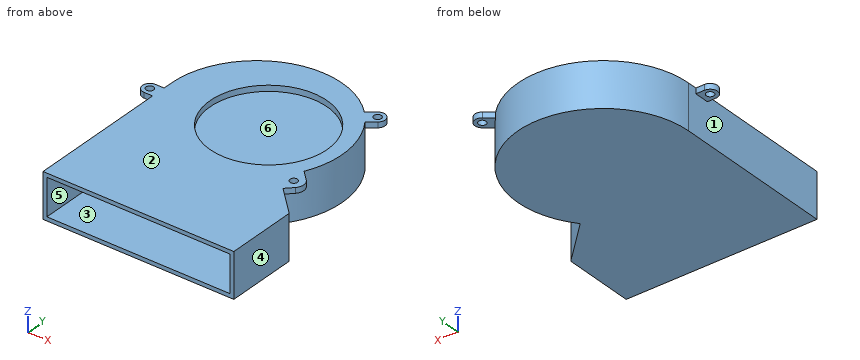
Autodesk Fusion 360 part; units mm, degrees
sketch "Esquisse1" plane through (0, 0, 0) normal (0, 0, 1) x (1, 0, 0)
  line L0 (0, 0) -> (98.3, 0)
  line L1 (98.3, 0) -> (98.3, 36.6)
  line L2 (98.3, 36.6) -> (77.8168, 56.6)
  arc A0 (77.8168, 56.6) -> (0, 84.75) centre (44, 84.75) ccw
  line L3 (0, 84.75) -> (0, 0)
  circle A1 centre (50.69, 84) radius 30.15
  point P0 (44, 128.75)
  point P1 (80.84, 84)
  point P2 (88, 84.75)
  point P3 (50.69, 114.15)
  dimension "d1" = 98.3
  dimension "d2" = 36.6
  dimension "d3" = 128.75
  dimension "d4" = 44
  dimension "d5" = 56.6
  dimension "d6" = 60.3
  dimension "d23" = 7.16
  dimension "d24" = 14.6
extrude "Extrusion1" add sketch "Esquisse1" along normal blind 23.06 contours L0 L1 L2 A0 L3 | A1
extrude "Extrusion2" cut sketch "Esquisse1" against normal blind 3 from surface at 23.06 contours A1
shell "Coque1" thickness 2 removed faces 1 at (32.7667, 0, 7.6867)
ref_plane "Plan de construction1" through (49.3725, 68.154, 23.06) normal (0, 0, 1) x (1, 0, 0)
sketch "Esquisse2" plane through (0, 0, 23.06) normal (0, 0, 1) x (1, 0, 0)
  circle A0 centre (84.6158, 57.1208) radius 1.95
  circle A1 centre (81.8543, 116.0561) radius 1.95
  circle A2 centre (-4.3677, 76.1716) radius 1.95
  line L0 (81.8543, 116.0561) -> (84.6158, 57.1208) construction
  line L1 (84.6158, 57.1208) -> (-4.3677, 76.1716) construction
  line L2 (81.8543, 116.0561) -> (-4.3677, 76.1716) construction
  circle A3 centre (44, 84.75) radius 49.1225 construction
  arc A4 (77.8168, 56.6) -> (0, 84.75) centre (44, 84.75) ccw construction
  circle A5 centre (84.6158, 57.1208) radius 5.1225
  line L3 (98.3, 36.6) -> (77.8168, 56.6) construction
  line L4 (84.7023, 49.877) -> (91.8596, 57.2072)
  line L5 (91.8596, 57.2072) -> (83.5013, 65.3684)
  line L6 (80.2019, 109.7584) -> (84.2761, 113.1278)
  arc A6 (84.2761, 113.1278) -> (79.4325, 118.9844) centre (81.8543, 116.0561) ccw
  line L7 (79.4325, 118.9844) -> (75.3584, 115.615)
  line L8 (0, 72.3716) -> (-4.3677, 72.3716)
  arc A7 (-4.3677, 79.9716) -> (-4.3677, 72.3716) centre (-4.3677, 76.1716) ccw
  line L9 (-4.3677, 79.9716) -> (0.2602, 79.9716)
  line L10 (81.8543, 116.0561) -> (44, 84.75) construction
  line L11 (44, 84.75) -> (84.6158, 57.1208) construction
  arc A8 (77.8168, 56.6) -> (0, 84.75) centre (44, 84.75) ccw
  line L12 (0, 84.75) -> (0, 0)
  line L13 (98.3, 36.6) -> (77.8168, 56.6)
  dimension "d15" = 3.9
  dimension "d16" = 59
  dimension "d17" = 95
  dimension "d18" = 91
  dimension "d19" = 7.6
  dimension "d20" = 7.6
extrude "Extrusion3" add sketch "Esquisse2" against normal blind 2.8 contours A5 | L8 A7 L9 L12 | L6 A6 L7 A8 | A5 L5 A8 | A5 L4 L13 | A5 A8 L13
equation "d4 = ( 88 / 2 ) * 1 mm"
equation "d20 = d19"
Verification items for the finished model (mm, model axes). Face numbers are marked on the shaded views. A direction names the side the tool comes from. Give positions to 0.01 mm unless a question says otherwise; leave off trailing zeros. Order: outer loops, then holes, each group sorted by start corner. A loop starts at its lowest first (then second) coordinate and runs counter-clockwise, first axis right, second up. Notation, with made-up numbers: M -24.5,-7.75 L 15.5,-7.75 A16 cw 15.5,21.25 Z; hole C 13,-21.5 d6. An arc over 180 degrees is marked long. Answer in a Markdown table with one row per item. Add a question column.
Item 1: Gauge pin test, flat ends, axial feed: pin 1 (8 mm diameter, centred on x = 83, y = 115.5, fed in from -Z); pin 2 (1.5 mm diameter, centred on y = 48.5, z = 4, fed in from -X); pin 3 (4 mm diameter, centred on y = 77, z = 4, fed in from +X). Record the tip position at first contact, or that the pin passes through.
Item 2: Section check D-D, the plane y = 89.5. Enter the section's corners in (x, z), and give its area (3 significant figures).
Item 3: Section check A-A, the plane y = 20. Enter the section's corners in (x, z).
Item 4: Mould release check, pull along Z, two halves, no side actions. Record for the marked faces 1, 2 and 3: released by +Z, released by -Z, zero draft, split by the parting line, or undercut.
Item 5: Tool access check on the marked faces 4, 5 and 6. Record the directions out of +Z, -Z, +X, -X, +Y, -Y that give a thin tool (end or side, any length) a straight path to the whole face; none if there is none.
Item 6: Section check B-B, the plane x = 65. Enter the section's corners in (y, z).
Item 7: Section check C-C, the plane z = 4. Enter the section's corners in (x, y).
Item 8: Scan lines: probe 1 along Z at (x, y) = (59.5, 9.5); probe 2 along Z at (x, y) = (65, 72); probe 3 along X at (y, z) = (23.5, 2.5). Record each from-to range of solid material in increasing order. Write a range as from..to.
Filled sheet:
| question | item | result |
|---|---|---|
| 1 | pin 1 | stops at z = 20.26 |
| 1 | pin 2 | stops at x = 0 |
| 1 | pin 3 | stops at x = 87.62 |
| 2 | outline | M 0.26,0 L 87.74,0 L 87.74,23.06 L 80.33,23.06 L 80.33,20.06 L 21.05,20.06 L 21.05,23.06 L 0.26,23.06 Z; hole M 2.27,2 L 85.73,2 L 85.73,21.06 L 82.37,21.06 L 82.37,18.06 L 19.01,18.06 L 19.01,21.06 L 2.27,21.06 Z |
| 2 | area | 439 mm^2 |
| 3 | outline | M 0,0 L 98.3,0 L 98.3,23.06 L 0,23.06 Z; hole M 2,2 L 96.3,2 L 96.3,21.06 L 2,21.06 Z |
| 4 | face 1 | zero draft |
| 4 | face 2 | released by +Z |
| 4 | face 3 | undercut |
| 5 | face 4 | +Z, -Z, +X, +Y, -Y |
| 5 | face 5 | -Y |
| 5 | face 6 | +Z |
| 6 | outline | M 0,0 L 123.42,0 L 123.42,23.06 L 110.54,23.06 L 110.54,20.06 L 57.46,20.06 L 57.46,23.06 L 0,23.06 L 0,21.06 L 55.21,21.06 L 55.21,18.06 L 112.79,18.06 L 112.79,21.06 L 121.12,21.06 L 121.12,2 L 0,2 Z |
| 7 | outline | M 0,0 L 2,0 L 2,84.75 A42 cw long 75.07,56.49 L 96.3,35.76 L 96.3,0 L 98.3,0 L 98.3,36.6 L 77.82,56.6 A44 ccw long 0,84.75 Z |
| 8 | probe 1 | z = 0..2, 21.06..23.06 |
| 8 | probe 2 | z = 0..2, 18.06..20.06 |
| 8 | probe 3 | x = 0..2, 96.3..98.3 |
